The listing builds one solid part. Answer for the finished solid, in the listing's coordinates (mm). A direction names the side the tool comes from. Round coordinates to 2 decimals unless told otherwise and drop trailing zeros. Loops run counter-clockwise (first coordinate to the right, second up) from the corner with the lowest first, then second, coordinate; pieces in that order, holes last. Notation, with made-up numbers: (51, 18) - (56, 18) arc R28 cw to (56, 41) - close; hole circle Ø1 at (8, 8). An arc over 180 degrees is marked (long way). Write item = value, one per line. Start each with the question number.
1) Given pin 1 Ø5 at (y, z) = (10.5, 24.5) entering from +X; pin 2 Ø8 at (x, z) = (-14, 29) entering from +Y; pin 3 Ø5 at (y, z) = (-3.5, -4) entering from -X, each flat-ended and moving along its own axis, determine where each tip first touches the part or whether it passes through.
2) Section A-A, the plane x = 0 is taken. Determine the outline of the cut face in (y, z).
3) For a pull along Z with two mould halves and no side action, classify faces 1 (the flat face through (0, 0, 40)), 2 (the cylindrical face through (-13.887, -10.648, 19.72)), 3 (the flat face through (2, -1, -7)) as released by +Z, released by -Z, zero draft, split by the parting line, or undercut.
4) Straight lines are drawn through the part: line 1 along Z through (x, y) = (13, -8.5); line 2 along Y through (x, z) = (12, 15); line 3 along Y through (x, z) = (-2.5, 5). For each, find the intervals that lie inside material, in ascending order.
5) Section D-D, the plane z = -12.5 is taken. Determine the outline of the cut face in (x, y).
6) A tool of negligible diameter and unlimited length cuts with its end or side. For faces 4 (the cylindrical face through (0.867, -3.905, -16.86)), 5 (the cylindrical face through (0, 2, -3)), 6 (the flat face through (0, 0, -27)), from which of +Z, -Z, +X, -X, +Y, -Y can it reach the whole face along a straight path? Write none if from no direction.
7) Section C-C, the plane z = 27.5 is taken. Determine the outline of the cut face in (x, y), and give its area (3 significant figures).
from build123d import *

# Parameters (mm, degrees)
SKETCH1_R                = 17.5
BOSS_EXTRUDE1_DEPTH      = 40
SKETCH2_R                = 2
BOSS_EXTRUDE2_DEPTH      = 17
BOSS_EXTRUDE3_DEPTH      = 10
BOSS_EXTRUDE3_DEPTH_BACK = 10
SKETCH3_R                = 4


with BuildPart() as part:
    # Sketch1 → Boss-Extrude1 (new body)
    with BuildSketch(Plane.XY):
        Circle(SKETCH1_R)
    extrude(amount=BOSS_EXTRUDE1_DEPTH)

    # Sketch2 → Boss-Extrude2 (add)
    with BuildSketch(Plane(origin=(0, 0, 0), x_dir=(-1, 0, 0), z_dir=(0, 0, -1))):
        with Locations(Location((0, 0, 0), (0, 0, 180))):
            Circle(SKETCH2_R)
    extrude(amount=BOSS_EXTRUDE2_DEPTH)

    # Sketch3 → Boss-Extrude3 (add, two sides: drawn at the far end of the back side and taken through both)
    with BuildSketch(Plane(origin=(0, 0, -17), x_dir=(-1, 0, 0), z_dir=(0, 0, -1)).offset(-BOSS_EXTRUDE3_DEPTH_BACK)):
        Circle(SKETCH3_R)
    extrude(amount=BOSS_EXTRUDE3_DEPTH + BOSS_EXTRUDE3_DEPTH_BACK)


solid = part.part
Geometry check:
q1.pin_1 = 15.56
q1.pin_2 = 14.36
q1.pin_3 = -1.73
q2.outline = (-17.5, 0) - (-2, 0) - (-2, -7) - (-4, -7) - (-4, -27) - (4, -27) - (4, -7) - (2, -7) - (2, 0) - (17.5, 0) - (17.5, 40) - (-17.5, 40) - close
q3.face_1 = released by +Z
q3.face_2 = zero draft
q3.face_3 = undercut
q4.line_1 = 0 to 40
q4.line_2 = -12.74 to 12.74
q4.line_3 = -17.32 to 17.32
q5.outline = circle Ø8 at (0, 0)
q6.face_4 = -Z
q6.face_5 = none
q6.face_6 = -Z, +X, -X, +Y, -Y
q7.outline = circle Ø35 at (0, 0)
q7.area = 962 mm2
